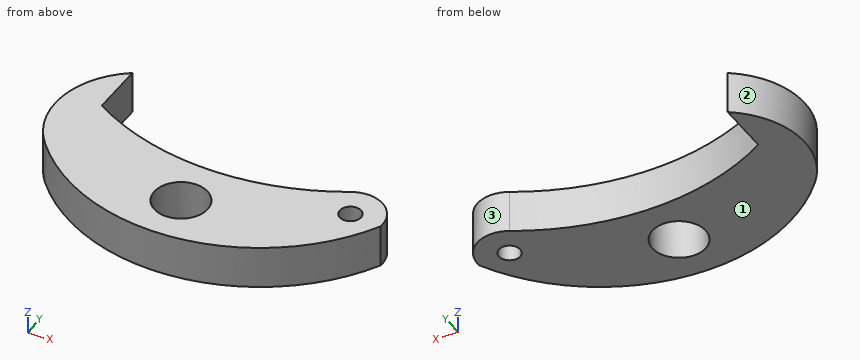
Autodesk Inventor part; units mm, degrees
ref_plane "YZ Plane" through (0, 0, 0) normal (1, 0, 0) x (0, 1, 0)
ref_plane "XZ Plane" through (0, 0, 0) normal (0, 1, 0) x (-1, 0, 0)
ref_plane "XY Plane" through (0, 0, 0) normal (0, 0, 1) x (1, 0, 0)
sketch "Sketch1" plane through (0, 0, 0) normal (0, 0, 1) x (1, 0, 0)
  circle A0 centre (0, 0) radius 1.25
  line L0 (-13.143, 0) -> (13.143, 0) construction
  line L1 (0, 15.5803) -> (0, -15.5803) construction
  circle A1 centre (6.5, 2.6) radius 0.5
  arc A2 (7.9939, 2.4651) -> (5.7614, 3.9055) centre (6.5, 2.6) ccw
  arc A3 (-6, 4.0443) -> (5.7614, 3.9055) centre (0, 14.0887) ccw
  line L2 (-6, 6.6) -> (-6, 4.0443)
  arc A4 (-6.75, 0.6471) -> (7.9939, 2.4651) centre (0, 6.6) ccw
  arc A5 (-6, 6.6) -> (-6.021, 0) centre (-3.75, 3.2928) ccw
  dimension "d0" = 2.6
  dimension "d1" = 6.5
  dimension "d2" = 1.5
  dimension "d3" = 1
  dimension "d4" = 2.5
  dimension "d5" = 11.7
  dimension "d6" = 6
  dimension "d7" = 9
  dimension "d8" = 6.6
  dimension "d10" = 6.6
  dimension "d11" = 4
extrude "Extrusion1" add sketch "Sketch1" along normal blind 2
properties part number "Hudson 1-66"
Verification items for the finished model (mm, model axes). Face numbers are marked on the shaded views. Coordinates: 2 decimals unless noted, no trailing zeros. Loops run counter-clockwise (first coordinate to the right, second up) from the corner with the lowest first, then second, coordinate; pieces in that order, holes last. Notation, with made-up numbers: M 58,31.5 L 117,31.5 A22 cw 117,53.5 Z; hole C -29,1 d1. An arc over 180 degrees is marked long. One line per item, written item: value.
1. Material ranges on line 1 along Y through (x, z) = (0, 1.05); line 2 along Y through (x, z) = (6.5, 1.55); line 3 along X through (y, z) = (0.25, 1.05), recorded low to high. Write a range as from..to.
Answers follow:
line 1: -2.4..-1.25, 1.25..2.39
line 2: 0.38..2.1, 3.1..4.1
line 3: -6.38..-1.22, 1.22..6.38
2. Section check C-C on z = 1.1. Record the cut outline in (x, y), plus the area to 3 significant figures.
Answers follow:
outline: M -6.75,0.65 A9 ccw 7.99,2.47 A1.5 ccw 5.76,3.91 A11.7 cw -6,4.04 L -6,6.6 A4 ccw Z; hole C 0,0 d2.5; hole C 6.5,2.6 d1
area: 63.4 mm^2
3. Section check D-D on x = -1.75. Record the cut outline in (y, z), plus the area to 3 significant figures.
Answers follow:
outline: M -2.23,0 L 2.52,0 L 2.52,2 L -2.23,2 Z
area: 9.50 mm^2
4. Section check A-A on x = 0. Record the cut outline in (y, z).
Answers follow:
outline: M -2.4,0 L -1.25,0 L -1.25,2 L -2.4,2 Z; M 1.25,0 L 2.39,0 L 2.39,2 L 1.25,2 Z
5. Mould release check, pull along X, two halves, no side actions. Record for the marked faces 1, 2 and 3: pulls with the +X half, pulls with the -X half, needs draft (parallel to the pull), parting line crosses it, or undercut.
Answers follow:
face 1: needs draft
face 2: pulls with the -X half
face 3: undercut
6. Section check B-B on y = 0. Record the cut outline in (x, z), plus the area to 3 significant figures.
Answers follow:
outline: M -6.12,0 L -1.25,0 L -1.25,2 L -6.12,2 Z; M 1.25,0 L 6.12,0 L 6.12,2 L 1.25,2 Z
area: 19.5 mm^2
7. Gauge pin test, flat ends, axial feed: P1, Ø1, axis at y = 5.5, z = 0.5, coming from the +X side; P2, Ø4, axis at x = 0, y = 0, coming from the -Z side. Record the tip position at first contact, or that the pin passes through.
Answers follow:
P1: x = -6
P2: z = 0
